Work out the finished part from the listing and answer in its coordinate system (mm). Face numbers are marked on the shaded views. Give positions to 0.01 mm unless a question says otherwise; leave off trailing zeros. Write each loop counter-clockwise with the first axis right and the second up, starting at its lowest first coordinate (ties: lowest second). Pieces come first, ordered by that corner, then holes.
1) Determine the mould class of the marked faces 1, 2 and 3 for opening direction X: pulls with the +X half, pulls with the -X half, needs draft (parallel to the pull), parting line crosses it, or undercut.
2) Given pin 1 Ø3.5 at (x, y) = (0, 8) entering from -Z, flat-ended and moving along its own axis, determine where the tip first touches the part or whether it passes through.
3) Find section D-D (z = -6.75). Determine the outline of the cut face in (x, y).
4) Straight lines are drawn through the part: probe 1 along Y at (x, z) = (0, -4.25); probe 2 along X at (y, z) = (-8, -4.5); probe 3 along Y at (x, z) = (1, -1.75). For each, find the intervals that lie inside material, in ascending order.
5) Find section C-C (y = 8). Determine the outline of the cut face in (x, z).
6) Find section B-B (x = 0). Determine the outline of the cut face in (y, z).
7) Find section A-A (z = -0.25). Determine the outline of the cut face in (x, y), plus the area to 3 significant figures.
Autodesk Inventor part; units mm, degrees
ref_plane "Work Plane1" through (-6, 0, 0) normal (1, 0, 0) x (0, 1, 0)
ref_plane "XZ Plane" through (0, 0, 0) normal (0, 1, 0) x (-1, 0, 0)
ref_plane "XY Plane" through (0, 0, 0) normal (0, 0, 1) x (1, 0, 0)
ref_plane "Work Plane1" through (-6, 0, 0) normal (1, 0, 0) x (0, 1, 0)
sketch "Sketch1" plane through (-6, 0, 0) normal (1, 0, 0) x (0, 1, 0)
  line L0 (-12, -8) -> (12, -8)
  arc A0 (-4, 0) -> (4, 0) centre (0, 0) ccw
  line L1 (-4, 0) -> (-12, 0)
  line L2 (12, -8) -> (12, 0)
  line L3 (-12, 0) -> (-12, -8)
  line L4 (12, 0) -> (4, 0)
extrude "Extrusion1" add sketch "Sketch1" along normal blind 12
hole "Hole2" at (0, -8, -8) direction (0, 0, 1) diameter 4.5 depth 8
sketch "Sketch2" plane through (-6, -12, -8) normal (0, 0, -1) x (-1, 0, 0)
  point P0 (-6, 4)
hole "Hole1" at (0, 8, -8) direction (0, 0, 1) diameter 4.5 depth 8
sketch "Sketch3" plane through (-6, -12, -8) normal (0, 0, -1) x (-1, 0, 0)
  point P0 (-6, 20)
properties part number "Hopper Smooth Rod Clamp" material "ASA Plastic"
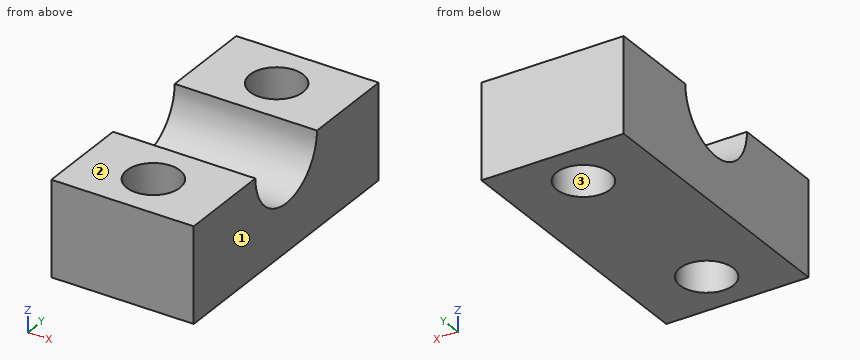
Results:
1. face 1: pulls with the +X half
1. face 2: needs draft
1. face 3: undercut
2. pin 1: passes through
3. outline: (-6, -12) - (6, -12) - (6, 12) - (-6, 12) - close; hole circle Ø4.5 at (0, -8); hole circle Ø4.5 at (0, 8)
4. probe 1: y = -12 to -10.25, -5.75 to 5.75, 10.25 to 12
4. probe 2: x = -6 to -2.25, 2.25 to 6
4. probe 3: y = -12 to -10.02, -5.98 to -3.6, 3.6 to 5.98, 10.02 to 12
5. outline: (-6, -8) - (-2.25, -8) - (-2.25, 0) - (-6, 0) - close; (2.25, -8) - (6, -8) - (6, 0) - (2.25, 0) - close
6. outline: (-12, -8) - (-10.25, -8) - (-10.25, 0) - (-12, 0) - close; (-5.75, -8) - (5.75, -8) - (5.75, 0) - (4, 0) arc R4 cw to (-4, 0) - (-5.75, 0) - close; (10.25, -8) - (12, -8) - (12, 0) - (10.25, 0) - close
7. outline: (-6, -12) - (6, -12) - (6, -3.99) - (-6, -3.99) - close; (-6, 3.99) - (6, 3.99) - (6, 12) - (-6, 12) - close; hole circle Ø4.5 at (0, -8); hole circle Ø4.5 at (0, 8)
7. area: 160 mm2
